Verification items for the finished model (mm, model axes). A direction names the side the tool comes from. Coordinates: 2 decimals unless noted, no trailing zeros. Order: outer loops, then holes, each group sorted by start corner. A loop starts at its lowest first (then second) coordinate and runs counter-clockwise, first axis right, second up.
Q1. Cross-section at A-A, the plane x = 37. Record the boundary of the cut face in (y, z).
Q2. Cross-section at D-D, the plane z = 16.5. Record the boundary of the cut face in (x, y).
Q3. Thickness scan on line 1 (Z direction, x = 23, y = -1.6); line 2 (Z direction, x = 45.6, y = 2.5); line 3 (Z direction, x = 18, y = 3.5). Record the ranges inside material, lowest first.
Q4. Cross-section at B-B, the plane y = 6.5. Count the separate pieces of the cut face and the enclosed holes in it, and give its area (3 significant figures).
Q5. Set-up check for faces 3 (the flat face through (44, 8, 16)), 4 (the flat face through (27, 7, 2)), 5 (the flat face through (16, -1, 5)): record each of +Z, -Z, +X, -X, +Y, -Y from which the full face is reachable in a straight line by a thin tool's end or side.
Q6. Cross-section at C-C, the plane x = 9. Record the boundary of the cut face in (y, z).
Q7. Depth check by flat-ended pin: P1, Ø5, axis at y = 4.5, z = 11.5, coming from the -X side; P2, Ø3, axis at y = 2.5, z = 4.5, coming from the -X side. Enter the tip coordinate at first touch or a pass-through.
Q8. Draft check along Z on faces 1 (the flat face through (0, 6, 17)), 2 (the flat face through (16, -1, 29)). Enter one of: pulls with the +Z half, pulls with the -Z half, needs draft (parallel to the pull), parting line crosses it, or undercut.
Autodesk Fusion 360 part; units mm, degrees
sketch "Skizze1" plane through (0, 0, 0) normal (0, 1, 0) x (1, 0, 0)
  line L0 (0, 0) -> (46, 0)
  line L1 (46, 0) -> (46, -33)
  line L2 (46, -33) -> (0, -33)
  line L3 (0, -33) -> (0, 0)
  line L4 (2, -2) -> (44, -2)
  line L5 (44, -2) -> (44, -31)
  line L6 (44, -31) -> (2, -31)
  line L7 (2, -31) -> (2, -2)
  dimension "d1" = 46
  dimension "d2" = 33
  dimension "d3" = 2
extrude "Extrusion1" add sketch "Skizze1" against normal blind 2 contours L0 L1 L2 L3 | L4 L5 L6 L7
extrude "Extrusion2" add sketch "Skizze1" along normal blind 15
sketch "Skizze2" plane through (0, 0, 0) normal (0, 1, 0) x (1, 0, 0)
sketch "Skizze3" plane through (0, 15, 0) normal (0, 1, 0) x (-1, 0, 0)
  line L0 (-44, 31) -> (-2, 31)
  line L1 (-2, 31) -> (-2, 2)
  line L2 (-2, 2) -> (-44, 2)
  line L3 (-44, 2) -> (-44, 31)
  line L4 (0, 33) -> (-46, 33)
  line L5 (-46, 33) -> (-46, 0)
  line L6 (-46, 0) -> (0, 0)
  line L7 (0, 0) -> (0, 33)
  line L8 (-2, 31) -> (-9.5, 31)
  line L9 (-9.5, 31) -> (-9.5, 2)
  line L10 (-9.5, 2) -> (-2, 2)
  line L11 (-2, 2) -> (-2, 31)
  dimension "d8" = 7.5
extrude "Extrusion3" add sketch "Skizze3" against normal blind 5 contours L0 L1 L2 L8 L9 L10 L11
sketch "Skizze4" plane through (0, -2, 0) normal (0, -1, 0) x (1, 0, 0)
  line L0 (46, 33) -> (0, 33)
  line L1 (0, 33) -> (0, 0)
  line L2 (0, 0) -> (46, 0)
  line L3 (46, 0) -> (46, 33)
  line L4 (46, 33) -> (16, 33)
  line L5 (16, 33) -> (16, 0)
  line L6 (16, 0) -> (46, 0)
  line L7 (46, 0) -> (46, 33)
  line L8 (16, 33) -> (46, 33)
  line L9 (16, 30) -> (16, 33)
  line L10 (16, 0) -> (46, 0)
  line L11 (46, 0) -> (46, 3)
  line L12 (46, 3) -> (16, 3)
  line L13 (16, 3) -> (16, 0)
  line L14 (16, 3) -> (46, 3)
  line L15 (46, 3) -> (46, 6)
  line L16 (46, 6) -> (16, 6)
  line L17 (16, 6) -> (16, 3)
  line L18 (0, 33) -> (46, 0)
  line L19 (46, 33) -> (0, 0)
  circle A0 centre (23, 16.5) radius 9.5
  line L20 (44, 35) -> (44, -3)
  line L21 (16, 30) -> (44, 30)
  line L22 (44, 30) -> (44, 27)
  line L23 (44, 27) -> (16, 27)
  line L24 (16, 27) -> (16, 30)
  dimension "d12" = 3
extrude "Extrusion4" cut sketch "Skizze4" against normal blind 6 contours L5 L19 L21 L23 L24 | L5 L18 A0 | L5 L18 L19 A0 | L19 L20 L21 L22 L23 | L5 L19 A0 | L5 L18 L19 | L5 L18 L19 A0 | L5 L12 L14 L16 L17 L18 | L5 L18 L19 A0 | L18 L19 A0 | L12 L14 L16 L18 L20
sketch "Skizze5" plane through (0, 0, 0) normal (0, 0, -1) x (1, 0, 0)
  line L0 (46, -15) -> (46, 2)
  line L1 (46, 2) -> (0, 2)
  line L2 (0, 2) -> (0, -15)
  line L3 (0, -15) -> (46, -15)
  line L4 (46, -15) -> (0, 2)
  line L5 (46, 2) -> (0, -15)
  circle A0 centre (23, -6.5) radius 3
  circle A1 centre (9, -6.5) radius 3
  circle A2 centre (37, -6.5) radius 3
  dimension "d17" = 14
  dimension "d18" = 0
  dimension "d21" = 6
extrude "Extrusion5" cut sketch "Skizze5" against normal blind 40 contours L4 L5 A0 | L4 L5 A0 | L4 L5 A0 | L4 L5 A0 | A1 | A2
sketch "Skizze6" plane through (0, 0, 0) normal (-1, 0, 0) x (0, -1, 0)
  line L0 (-15, 0) -> (2, 0)
  line L1 (2, 0) -> (2, 33)
  line L2 (2, 33) -> (-15, 33)
  line L3 (-15, 33) -> (-15, 0)
  line L4 (-15, 33) -> (2, 0)
  circle A0 centre (-6.5, 16.5) radius 2
  circle A1 centre (-2.5, 16.5) radius 2
  circle A2 centre (-2.5, 4.5) radius 2
  circle A3 centre (-2.5, 10.5) radius 2
  circle A4 centre (-2.5, 22.5) radius 2
  circle A5 centre (-2.5, 28.5) radius 2
  dimension "d22" = 4
  dimension "d25" = 4
  dimension "d26" = 0
  dimension "d29" = 0
  dimension "d30" = 12
extrude "Extrusion6" cut sketch "Skizze6" against normal blind 130 contours A1 | L4 A2 | L4 A2 | L4 A3 | L4 A3 | A4 | A5
Check values:
1. outline: (-2, 0) - (3.5, 0) - (3.5, 2) - (0, 2) - (0, 3) - (-2, 3) - close; (-2, 6) - (0, 6) - (0, 27) - (-2, 27) - close; (-2, 30) - (0, 30) - (0, 31) - (3.5, 31) - (3.5, 33) - (-2, 33) - close; (9.5, 0) - (15, 0) - (15, 2) - (9.5, 2) - close; (9.5, 31) - (15, 31) - (15, 33) - (9.5, 33) - close
2. outline: (0, -2) - (13.5, -2) - (13.5, 0) - (2, 0) - (2, 0.5) - (0, 0.5) - close; (0, 4.5) - (2, 4.5) - (2, 10) - (9.5, 10) - (9.5, 15) - (0, 15) - close; (32.5, -2) - (46, -2) - (46, 0.5) - (44, 0.5) - (44, 0) - (32.5, 0) - close; (44, 4.5) - (46, 4.5) - (46, 15) - (44, 15) - close
3. line 1: z = 0 to 3, 6 to 7, 26 to 27, 30 to 33
3. line 2: z = 0 to 2.5, 6.5 to 8.5, 12.5 to 14.5, 18.5 to 20.5, 24.5 to 26.5, 30.5 to 33
3. line 3: z = 0 to 2, 31 to 33
4. separate pieces: 6
4. enclosed holes: 0
4. area: 228 mm2
5. face 3: +Y
5. face 4: none
5. face 5: +Y, -Y
6. outline: (-2, 0) - (3.5, 0) - (3.5, 2) - (0, 2) - (0, 31) - (3.5, 31) - (3.5, 33) - (-2, 33) - close; (9.5, 0) - (15, 0) - (15, 33) - (9.5, 33) - (9.5, 31) - (10, 31) - (10, 2) - (9.5, 2) - close
7. P1: stops at x = 0
7. P2: passes through
8. face 1: needs draft
8. face 2: undercut
